```python
from build123d import *

# Parameters (mm, degrees)
F0_W        = 39
F0_H        = 39
F0_R        = 16.5
F1_DEPTH    = 90
F0_R_2      = 2
F2_DEPTH    = 3
F3_W        = 75
F3_H        = 23
F4_DEPTH    = 21.5
F5_DEPTH    = 10
F6_T1_DEPTH = 127.5
F6_T3_DEPTH = 40.5


# Not quite as in the source:
# - a fillet or chamfer that OpenCascade refuses, or shapes differently, is made with other operations: its cross-section is extruded or revolved along the edge and cut away or added
# - a feature names something its author has since deleted; it is built from what else it names


with BuildPart() as f1:
    # F0 (on Right) → F1 (new body)
    with BuildSketch(Plane.YZ):
        with Locations((0, 2)):
            Rectangle(F0_W, F0_H)
        Circle(F0_R, mode=Mode.SUBTRACT)
        Circle(F0_R)
        with BuildLine():
            ThreePointArc((5.25, 13.5161939909), (11.9660979438, 8.1891696771), (14.5, 0))
            ThreePointArc((14.5, 0), (11.9660979438, -8.1891696771), (5.25, -13.5161939909))
            ThreePointArc((5.25, -13.5161939909), (0, -14.5), (-5.25, -13.5161939909))
            ThreePointArc((-5.25, -13.5161939909), (-14.5, 0), (-5.25, 13.5161939909))
            ThreePointArc((-5.25, 13.5161939909), (0, 14.5), (5.25, 13.5161939909))
        make_face(mode=Mode.SUBTRACT)
    extrude(amount=-F1_DEPTH)

    # F0 (on Right) → F2 (join)
    with BuildSketch(Plane.YZ):
        with Locations((0, 2)):
            Rectangle(F0_W, F0_H)
        Circle(F0_R, mode=Mode.SUBTRACT)
        Circle(F0_R)
        with BuildLine():
            ThreePointArc((5.25, 13.5161939909), (11.9660979438, 8.1891696771), (14.5, 0))
            ThreePointArc((14.5, 0), (11.9660979438, -8.1891696771), (5.25, -13.5161939909))
            ThreePointArc((5.25, -13.5161939909), (0, -14.5), (-5.25, -13.5161939909))
            ThreePointArc((-5.25, -13.5161939909), (-14.5, 0), (-5.25, 13.5161939909))
            ThreePointArc((-5.25, 13.5161939909), (0, 14.5), (5.25, 13.5161939909))
        make_face(mode=Mode.SUBTRACT)
        with BuildLine():
            ThreePointArc((5.25, -13.5161939909), (11.9660979438, -8.1891696771), (14.5, 0))
            ThreePointArc((14.5, 0), (11.9660979438, 8.1891696771), (5.25, 13.5161939909))
            Line((5.25, 13.5161939909), (5.25, 8.5))
            Line((5.25, 8.5), (-5.25, 8.5))
            Line((-5.25, 8.5), (-5.25, 13.5161939909))
            ThreePointArc((-5.25, 13.5161939909), (-14.5, 0), (-5.25, -13.5161939909))
            Line((-5.25, -13.5161939909), (-5.25, -8.5))
            Line((-5.25, -8.5), (5.25, -8.5))
            Line((5.25, -8.5), (5.25, -13.5161939909))
        make_face()
        Circle(F0_R_2, mode=Mode.SUBTRACT)
        Circle(F0_R_2)
    extrude(amount=F2_DEPTH)

    # F3 (on face) → F4 (cut)
    with BuildSketch(Plane(origin=(0, 0, -17.5), x_dir=(1, 0, 0), z_dir=(0, 0, -1))):
        with Locations((-44.5, 0)):
            Rectangle(F3_W, F3_H)
    extrude(amount=-F4_DEPTH, mode=Mode.SUBTRACT)

    # F0 (on Right) → F5 (join)
    with BuildSketch(Plane.YZ):
        Circle(F0_R_2)
    extrude(amount=-F5_DEPTH)

    # F6: fillet of radius 15 on 8 edges, made by hand

    # F6_s2 → F6_t1 (cut)
    with BuildSketch(Plane.YZ.offset(-127.5)):
        with BuildLine():
            ThreePointArc((4.5, -17.5), (15.1066017178, -13.1066017178), (19.5, -2.5))
            Line((19.5, -2.5), (19.5, -17.5))
            Line((19.5, -17.5), (4.5, -17.5))
        make_face()
        with BuildLine():
            ThreePointArc((-19.5, -2.5), (-15.1066017178, -13.1066017178), (-4.5, -17.5))
            Line((-4.5, -17.5), (-19.5, -17.5))
            Line((-19.5, -17.5), (-19.5, -2.5))
        make_face()
        with BuildLine():
            ThreePointArc((4.5, 21.5), (15.1066017178, 17.1066017178), (19.5, 6.5))
            Line((19.5, 6.5), (19.5, 21.5))
            Line((19.5, 21.5), (4.5, 21.5))
        make_face()
        with BuildLine():
            ThreePointArc((-4.5, 21.5), (-15.1066017178, 17.1066017178), (-19.5, 6.5))
            Line((-19.5, 6.5), (-19.5, 21.5))
            Line((-19.5, 21.5), (-4.5, 21.5))
        make_face()
    extrude(amount=F6_T1_DEPTH, mode=Mode.SUBTRACT)

    # F6_s4 → F6_t3 (cut)
    with BuildSketch(Plane.YZ):
        with BuildLine():
            ThreePointArc((4.5, -17.5), (15.1066017178, -13.1066017178), (19.5, -2.5))
            Line((19.5, -2.5), (19.5, -17.5))
            Line((19.5, -17.5), (4.5, -17.5))
        make_face()
        with BuildLine():
            ThreePointArc((-19.5, -2.5), (-15.1066017178, -13.1066017178), (-4.5, -17.5))
            Line((-4.5, -17.5), (-19.5, -17.5))
            Line((-19.5, -17.5), (-19.5, -2.5))
        make_face()
        with BuildLine():
            ThreePointArc((4.5, 21.5), (15.1066017178, 17.1066017178), (19.5, 6.5))
            Line((19.5, 6.5), (19.5, 21.5))
            Line((19.5, 21.5), (4.5, 21.5))
        make_face()
        with BuildLine():
            ThreePointArc((-4.5, 21.5), (-15.1066017178, 17.1066017178), (-19.5, 6.5))
            Line((-19.5, 6.5), (-19.5, 21.5))
            Line((-19.5, 21.5), (-4.5, 21.5))
        make_face()
    extrude(amount=F6_T3_DEPTH, mode=Mode.SUBTRACT)


solid = f1.part
```
Design review of the part built by this model. Coordinates are the model's own, in mm. A direction names the side the tool comes from. Coordinates: 2 decimals unless noted, no trailing zeros. Order: outer loops, then holes, each group sorted by start corner. A loop starts at its lowest first (then second) coordinate and runs counter-clockwise, first axis right, second up. Notation, with made-up numbers: (69, -9) -> (83, -9) arc R14 ccw to (83, 12) -> close; hole circle Ø9 at (-37.5, 7). An arc over 180 degrees is marked (long way). One line per item, written item: value. Start each with the question number.
Q1. Tool access review of faces 1 (the flat face through (-45, 11.5, -12)), 2 (the flat face through (0, 0, 3)), 3 (the flat face through (1, -5.25, 11)), 4 (the cylindrical face through (-44.15, -14.99, 17.22)), 5 (the flat face through (-10, 0, 0)): name each direction out of +Z, -Z, +X, -X, +Y, -Y from which nothing blocks a thin tool from reaching the whole face with its end or side.
Q2. Take a section at C-C, the plane y = 10.5. State the section outline as (x, z) points.
Q3. Take a section at B-B, the plane x = -20.5. State the section outline as (y, z) points.
Q4. Take a section at D-D, the plane z = -3.5. State the section outline as (x, y) points.
Q5. For probe 1 along X at (y, z) = (12, -4.5); probe 2 along Y at (x, z) = (-29, -13.5); probe 3 along Y at (x, z) = (-67, -5), list the stretches that pass through material, from the lowest coordinate up.
Q6. Insertion check: pin 1 Ø7 at (y, z) = (1.5, -13) entering from +X; pin 2 Ø0.9 at (x, z) = (1.5, 11) entering from -Y; pin 3 Ø13.5 at (y, z) = (-4.5, -1) entering from -X; pin 4 Ø3 at (x, z) = (-47, 12) entering from +Y. Each pin has a flat end and moves straight along its axis. Give the tip position at first contact, or say it passes through.
Q7. Mouldability with a two-part tool opening along Y and no side actions: class faces 6 (the flat face through (-7, 0, -15)), 7 (the flat face through (-2, 0, -17.5)), 8 (the flat face through (-44, 19.5, 2)), 9 (the flat face through (1, 0, -8.5)) as pulls with the +Y half, pulls with the -Y half, needs draft (parallel to the pull), parting line crosses it, or undercut.
Q8. Take a section at A-A, the plane y = 0. State the section outline as (x, z) points, then the cut area to 3 significant figures.
Values follow:
1. face 1: -Z
1. face 2: -X
1. face 3: +X, -X
1. face 4: +Z, +X, -X, -Y
1. face 5: -Z, -X
2. outline: (-90, -16.25) -> (-82, -16.25) -> (-82, -10) -> (-90, -10) -> close; (-90, 10) -> (0, 10) -> (0, -10) -> (-7, -10) -> (-7, -16.25) -> (3, -16.25) -> (3, 20.25) -> (-90, 20.25) -> close
3. outline: (-19.5, -2.5) arc R15 ccw to (-11.5, -15.77) -> (-11.5, -8.83) arc R14.5 cw (long way) to (11.5, -8.83) -> (11.5, -15.77) arc R15 ccw to (19.5, -2.5) -> (19.5, 6.5) arc R15 ccw to (4.5, 21.5) -> (-4.5, 21.5) arc R15 ccw to (-19.5, 6.5) -> close
4. outline: (-90, -19.47) -> (3, -19.47) -> (3, 19.47) -> (-90, 19.47) -> (-90, 14.07) -> (0, 14.07) -> (0, -14.07) -> (-90, -14.07) -> close
5. probe 1: x = 0 to 3
5. probe 2: y = -14.7 to -11.5, 11.5 to 14.7
5. probe 3: y = -19.29 to -13.61, 13.61 to 19.29
6. pin 1: stops at x = 3
6. pin 2: stops at y = -18.94
6. pin 3: stops at x = -10
6. pin 4: stops at y = 18.96
7. face 6: undercut
7. face 7: needs draft
7. face 8: pulls with the +Y half
7. face 9: undercut
8. outline: (-90, -17.5) -> (-82, -17.5) -> (-82, -14.5) -> (-90, -14.5) -> close; (-90, 14.5) -> (3, 14.5) -> (3, 21.5) -> (-90, 21.5) -> close; (-10, -2) -> (0, -2) -> (0, -8.5) -> (3, -8.5) -> (3, 8.5) -> (0, 8.5) -> (0, 2) -> (-10, 2) -> close; (-7, -17.5) -> (3, -17.5) -> (3, -14.5) -> (-7, -14.5) -> close
8. area: 796 mm2
